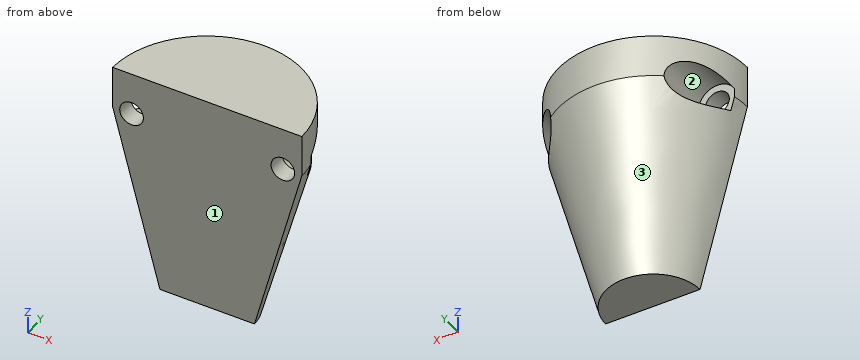
from build123d import *

# Parameters (mm, degrees)
SKETCH1_R           = 12.7
BOSS_EXTRUDE1_DEPTH = 58.7248
CHAMFER3_SIZE       = 6.35
CHAMFER3_SIZE2      = 23.698522628
CHAMFER4_SIZE       = 6.35
CHAMFER4_SIZE2      = 23.698522628
CUT_EXTRUDE1_DEPTH  = 58.7248
CUT_EXTRUDE2_DEPTH  = 58.7248
CUT_EXTRUDE3_DEPTH  = 35.419680486
SKETCH5_R           = 1.5875
CUT_EXTRUDE4_DEPTH  = 62.383681342
SKETCH6_R           = 2.54
CUT_EXTRUDE5_DEPTH  = 10.16


with BuildPart() as part:
    # Sketch1 → Boss-Extrude1 (new body)
    with BuildSketch(Plane.XY):
        Circle(SKETCH1_R)
    extrude(amount=-BOSS_EXTRUDE1_DEPTH)

    # Chamfer3
    chamfer3_edges = [part.edges().sort_by_distance(p)[0] for p in [
        (-12.7, 0, -58.7248),
    ]]
    chamfer3_side = [part.faces().sort_by_distance(p)[0] for p in [
        (0, 0, -58.7248),
    ]]
    chamfer(chamfer3_edges, length=CHAMFER3_SIZE, length2=CHAMFER3_SIZE2, reference=chamfer3_side[0])

    # Chamfer4
    chamfer4_edges = [part.edges().sort_by_distance(p)[0] for p in [
        (-12.7, 0, 0),
    ]]
    chamfer4_side = [part.faces().sort_by_distance(p)[0] for p in [
        (0, 0, 0),
    ]]
    chamfer(chamfer4_edges, length=CHAMFER4_SIZE, length2=CHAMFER4_SIZE2, reference=chamfer4_side[0])

    # Sketch2 → Cut-Extrude1 (cut)
    with BuildSketch(Plane(origin=(0, 0, 0), x_dir=(1, 0, 0), z_dir=(0, 1, 0))):
        Polygon((-6.35, 0), (-12.7, 23.698522628), (-12.7, 35.026277372), (-6.35, 58.7248), (6.35, 58.7248), (12.7, 35.026277372), (12.7, 23.698522628), (6.35, 0), align=None)
    extrude(amount=-CUT_EXTRUDE1_DEPTH, mode=Mode.SUBTRACT)

    # Sketch3 → Cut-Extrude2 (cut)
    with BuildSketch(Plane.XY):
        with BuildLine():
            Line((-12.7, 0), (12.7, 0))
            ThreePointArc((12.7, 0), (12.699841245, 0.063500794), (12.699364984, 0.127))
            Line((12.699364984, 0.127), (0, 0.127))
            Line((0, 0.127), (-12.699364984, 0.127))
            ThreePointArc((-12.699364984, 0.127), (-12.699841245, 0.063500794), (-12.7, 0))
        make_face()
    extrude(amount=-CUT_EXTRUDE2_DEPTH, mode=Mode.SUBTRACT)

    # Sketch4 → Cut-Extrude3 (cut, through all)
    with BuildSketch(Plane(origin=(0, 0, -29.3624), x_dir=(-1, 0, 0), z_dir=(0, 0, -1))):
        with BuildLine():
            Line((0, 0.127), (-12.699364984, 0.127))
            ThreePointArc((-12.699364984, 0.127), (0, 12.826364984), (12.699364984, 0.127))
            Line((12.699364984, 0.127), (0, 0.127))
        make_face()
    extrude(amount=-CUT_EXTRUDE3_DEPTH, mode=Mode.SUBTRACT)

    # Sketch5 → Cut-Extrude4 (cut, through all)
    with BuildSketch(Plane(origin=(0, 12.7, 0), x_dir=(-1, 0, 0), z_dir=(0, -1, 0))):
        with Locations((-10.16, 35.026277372)):
            Circle(SKETCH5_R)
        with Locations(Location((10.16, 35.026277372, 0), (0, 0, 270))):
            Circle(SKETCH5_R)
    extrude(amount=CUT_EXTRUDE4_DEPTH, mode=Mode.SUBTRACT)

    # Sketch6 → Cut-Extrude5 (cut)
    with BuildSketch(Plane(origin=(0, 12.7, 0), x_dir=(-1, 0, 0), z_dir=(0, -1, 0))):
        with Locations((-10.16, 35.026277372)):
            Circle(SKETCH6_R)
        with Locations((10.16, 35.026277372)):
            Circle(SKETCH6_R)
    extrude(amount=CUT_EXTRUDE5_DEPTH, mode=Mode.SUBTRACT)


solid = part.part
The model under review builds one solid part; all positions refer to its coordinate system, in mm. Face numbers are marked on the shaded views. Round coordinates to 2 decimals unless told otherwise and drop trailing zeros. Loops run counter-clockwise (first coordinate to the right, second up) from the corner with the lowest first, then second, coordinate; pieces in that order, holes last. Notation, with made-up numbers: (-13.5, -3.75) -> (6.5, -3.75) arc R28 cw to (6.5, 24.25) -> close; hole circle Ø4 at (49.25, -25.75). An arc over 180 degrees is marked (long way). One line per question, with ' | ' between items. Start each with the question number.
Item 1: Wall thickness on line 1 along X through (y, z) = (2.5, -34.5); line 2 along X through (y, z) = (9.75, -32); line 3 along Y through (x, z) = (2, -46): over which ranges is each line inside the solid? List them lowest first. Write a range as [from, to].
Item 2: Draft analysis for pull direction X (two halves, no side actions). For the marked faces 1, 2 and 3, state which applies: +X half, -X half, draft (parallel to the pull), parting line (faces both ways), or undercut.
Item 3: For pin 1 (5.5 mm diameter, centred on x = -10, z = -34.5, fed in from +Y); pin 2 (1 mm diameter, centred on y = 8, z = -50.5, fed in from +X); pin 3 (5 mm diameter, centred on y = 10, z = -48.5, fed in from -X), all flat-tipped, find the tip position at first contact; note any pin that passes through.
Item 4: Add section A-A, the plane x = 0. Write out the cut boundary in (y, z), then the cut area to 3 significant figures.
Return value:
1) line 1: x = [-12.45, -11.66], [-8.66, 8.66], [11.66, 12.45] | line 2: x = [-8.14, 8.14] | line 3: y = [0.13, 9.55]
2) face 1: draft | face 2: undercut | face 3: parting line
3) pin 1: stops at y = 10.43 | pin 2: stops at x = 4.15 | pin 3: stops at x = -5.32
4) outline: (0.13, -58.72) -> (6.35, -58.72) -> (12.7, -35.03) -> (12.7, -29.36) -> (0.13, -29.36) -> close | area: 294 mm2
